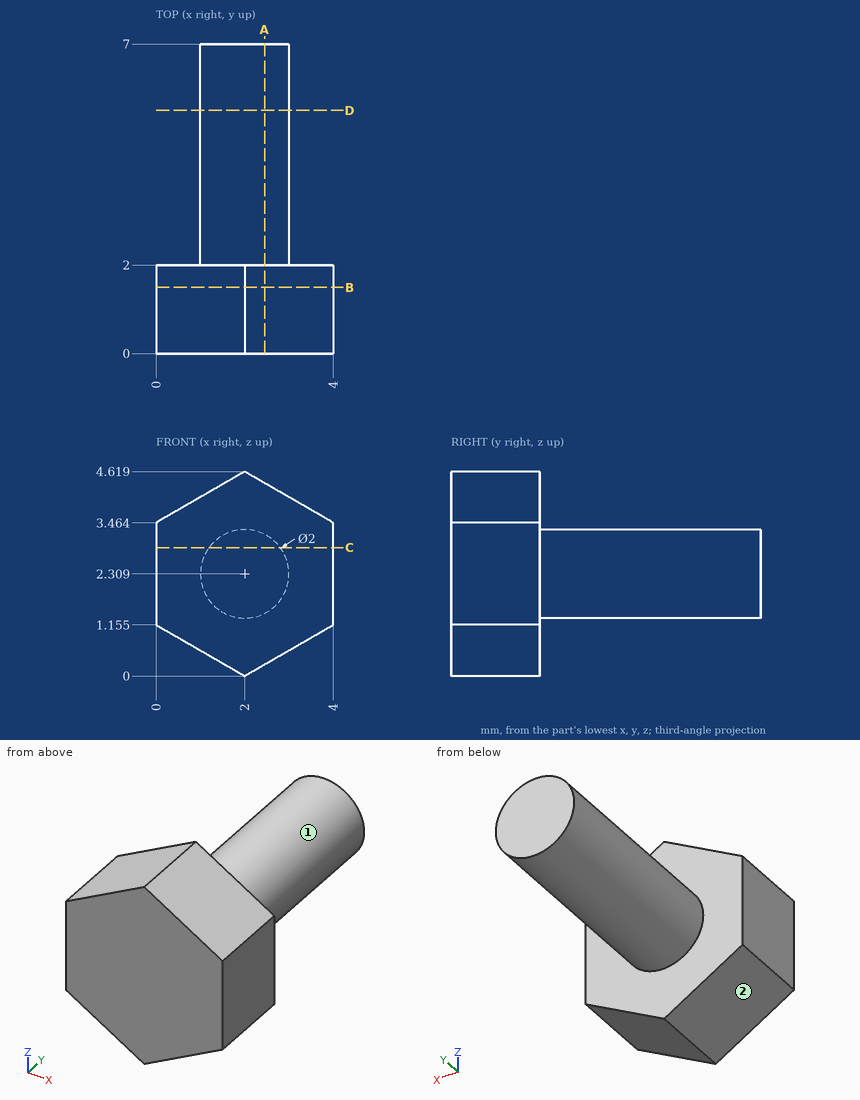
The drawing under review shows one solid part. Ordinate dimensions are in mm from its lowest x, y, z. A direction names the side the tool comes from. Coordinates: 2 decimals unless noted, no trailing zeros. Loops run counter-clockwise (first coordinate to the right, second up) from the corner with the lowest first, then second, coordinate; pieces in that order, holes last. Notation, with made-up numbers: (39, 11) -> (45, 11) arc R25 ccw to (45, 36) -> close; hole circle Ø1 at (53.25, 71). An arc over 180 degrees is marked (long way). Answer as a JSON object with one key per item and string values.
Q1. Take a section at D-D on y = 5.5. Give the boundary of the cut face in (x, z).
Answer block:
{"outline": "circle Ø2 at (2, 2.31)"}
Q2. Clearance check with a flat-ended pin moving along its axis: pin 1 Ø1.5 at (x, y) = (3, 3.5) entering from +Z. State where the tip first meets the part, or that it passes through.
Answer block:
{"pin 1": "stops at z = 3.28"}
Q3. Take a section at A-A on x = 2.45. Give the boundary of the cut face in (y, z), plus the area to 3 significant figures.
Answer block:
{"outline": "(0, 0.26) -> (2, 0.26) -> (2, 1.42) -> (7, 1.42) -> (7, 3.2) -> (2, 3.2) -> (2, 4.36) -> (0, 4.36) -> close", "area": "17.1 mm^2"}
Q4. Tool access review of the marked faces 1 and 2: name each direction out of +Z, -Z, +X, -X, +Y, -Y from which nothing blocks a thin tool from reaching the whole face with its end or side.
Answer block:
{"face 1": "+Y", "face 2": "-Z, -X, +Y, -Y"}
Q5. Take a section at C-C on z = 2.9. Give the boundary of the cut face in (x, y).
Answer block:
{"outline": "(0, 0) -> (4, 0) -> (4, 2) -> (2.81, 2) -> (2.81, 7) -> (1.19, 7) -> (1.19, 2) -> (0, 2) -> close"}
Q6. Take a section at B-B on y = 1.5. Give the boundary of the cut face in (x, z) (1 decimal).
Answer block:
{"outline": "(0, 1.2) -> (2, 0) -> (4, 1.2) -> (4, 3.5) -> (2, 4.6) -> (0, 3.5) -> close"}
Q7. To check wall thickness, follow L1, parallel to Y at x = 3.55, z = 1.2; L2, parallel to X at y = 2.5, z = 2.25; L3, parallel to Z at x = 2.8, y = 1.5. State the ranges of each line that lie inside material, in increasing order.
Answer block:
{"L1": "y = 0 to 2", "L2": "x = 1 to 3", "L3": "z = 0.46 to 4.16"}
